Geometry check sheet. Reference: the model listing, model coordinates, mm. Give positions to 0.01 mm unless a question says otherwise; leave off trailing zeros. Answer as CSV lines item,"result".
from build123d import *

# Parameters (mm, degrees)
F0_W     = 1240
F0_H     = 655
F0_W_2   = 1200
F0_H_2   = 600
F1_DEPTH = 40
F3_DEPTH = 600
F4_R     = 7.5
F5_DEPTH = 600
F6_W     = 1240
F6_H     = 655
F6_W_2   = 1200
F6_H_2   = 600
F7_DEPTH = 40


with BuildPart() as f1:
    # F0 (on Top) → F1 (new body)
    with BuildSketch(Plane.XY):
        Rectangle(F0_W, F0_H)
        Rectangle(F0_W_2, F0_H_2, mode=Mode.SUBTRACT)
    extrude(amount=F1_DEPTH)

    # F2 (on face) → F3 (join)
    with BuildSketch(Plane.XY.offset(40)):
        Polygon((-600, 327.5), (-620, 327.5), (-620, 277.5), (-600, 277.5), (-600, 300), align=None)
        Polygon((-600, -277.5), (-620, -277.5), (-620, -327.5), (-600, -327.5), (-600, -300), align=None)
        Polygon((620, 327.5), (600, 327.5), (600, 300), (600, 277.5), (620, 277.5), align=None)
        Polygon((620, -277.5), (600, -277.5), (600, -300), (600, -327.5), (620, -327.5), align=None)
    extrude(amount=F3_DEPTH)

    # F4 (on face) → F5 (join)
    with BuildSketch(Plane.XY.offset(40)):
        with Locations((-550, -315)):
            Circle(F4_R)
        with Locations((-500, -315)):
            Circle(F4_R)
        with Locations((-450, -315)):
            Circle(F4_R)
        with Locations((-400, -315)):
            Circle(F4_R)
        with Locations((-350, -315)):
            Circle(F4_R)
        with Locations((-300, -315)):
            Circle(F4_R)
        with Locations((-250, -315)):
            Circle(F4_R)
        with Locations((-200, -315)):
            Circle(F4_R)
        with Locations((-150, -315)):
            Circle(F4_R)
        with Locations((-100, -315)):
            Circle(F4_R)
        with Locations((-50, -315)):
            Circle(F4_R)
        with Locations((0, -315)):
            Circle(F4_R)
        with Locations((50, -315)):
            Circle(F4_R)
        with Locations((100, -315)):
            Circle(F4_R)
        with Locations((150, -315)):
            Circle(F4_R)
        with Locations((200, -315)):
            Circle(F4_R)
        with Locations((250, -315)):
            Circle(F4_R)
        with Locations((300, -315)):
            Circle(F4_R)
        with Locations((350, -315)):
            Circle(F4_R)
        with Locations((400, -315)):
            Circle(F4_R)
        with Locations((450, -315)):
            Circle(F4_R)
        with Locations((500, -315)):
            Circle(F4_R)
        with Locations((550, -315)):
            Circle(F4_R)
        with Locations((-500, 315)):
            Circle(F4_R)
        with Locations((-550, 315)):
            Circle(F4_R)
        with Locations((150, 315)):
            Circle(F4_R)
        with Locations((0, 315)):
            Circle(F4_R)
        with Locations((250, 315)):
            Circle(F4_R)
        with Locations((-400, 315)):
            Circle(F4_R)
        with Locations((450, 315)):
            Circle(F4_R)
        with Locations((100, 315)):
            Circle(F4_R)
        with Locations((500, 315)):
            Circle(F4_R)
        with Locations((-100, 315)):
            Circle(F4_R)
        with Locations((-450, 315)):
            Circle(F4_R)
        with Locations((400, 315)):
            Circle(F4_R)
        with Locations((50, 315)):
            Circle(F4_R)
        with Locations((-300, 315)):
            Circle(F4_R)
        with Locations((-50, 315)):
            Circle(F4_R)
        with Locations((550, 315)):
            Circle(F4_R)
        with Locations((300, 315)):
            Circle(F4_R)
        with Locations((-200, 315)):
            Circle(F4_R)
        with Locations((200, 315)):
            Circle(F4_R)
        with Locations((350, 315)):
            Circle(F4_R)
        with Locations((-250, 315)):
            Circle(F4_R)
        with Locations((-150, 315)):
            Circle(F4_R)
        with Locations((-350, 315)):
            Circle(F4_R)
        with Locations((-610, -263.75)):
            Circle(F4_R)
        with Locations((-610, -213.75)):
            Circle(F4_R)
        with Locations((-610, -163.75)):
            Circle(F4_R)
        with Locations((-610, -113.75)):
            Circle(F4_R)
        with Locations((-610, -63.75)):
            Circle(F4_R)
        with Locations((-610, -13.75)):
            Circle(F4_R)
        with Locations((-610, 36.25)):
            Circle(F4_R)
        with Locations((-610, 86.25)):
            Circle(F4_R)
        with Locations((-610, 136.25)):
            Circle(F4_R)
        with Locations((-610, 186.25)):
            Circle(F4_R)
        with Locations((-610, 236.25)):
            Circle(F4_R)
        with Locations((610, -263.75)):
            Circle(F4_R)
        with Locations((610, -213.75)):
            Circle(F4_R)
        with Locations((610, 136.25)):
            Circle(F4_R)
        with Locations((610, 236.25)):
            Circle(F4_R)
        with Locations((610, -113.75)):
            Circle(F4_R)
        with Locations((610, 86.25)):
            Circle(F4_R)
        with Locations((610, 186.25)):
            Circle(F4_R)
        with Locations((610, 36.25)):
            Circle(F4_R)
        with Locations((610, -13.75)):
            Circle(F4_R)
        with Locations((610, -63.75)):
            Circle(F4_R)
        with Locations((610, -163.75)):
            Circle(F4_R)
    extrude(amount=F5_DEPTH)

    # F6 (on face) → F7 (join)
    with BuildSketch(Plane.XY.offset(640)):
        Rectangle(F6_W, F6_H)
        Rectangle(F6_W_2, F6_H_2, mode=Mode.SUBTRACT)
    extrude(amount=F7_DEPTH)


solid = f1.part
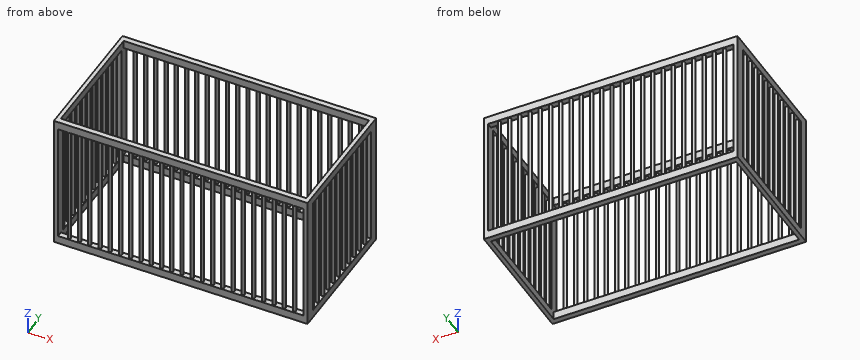
(1) Material ranges on line 1 (Y direction, x = 1.5, z = 130); line 2 (Y direction, x = 145, z = 653.5); line 3 (X direction, y = -287.5, z = 560.5), recorded low to high.
The answers:
line 1,"y = -322.35 to -307.65, 307.65 to 322.35"
line 2,"y = -327.5 to -300, 300 to 327.5"
line 3,"x = -620 to -600, 600 to 620"
(2) Section check A-A on z = 380.5. State how many separate pieces and enclosed holes the cut face has, then the cut area to 3 significant figures.
The answers:
separate pieces,"72"
enclosed holes,"0"
area,"16,000 mm2"
(3) Gauge pin test, flat ends, axial feed: P1, Ø8, axis at y = 182.5, z = 220.5, coming from the -X side; P2, Ø6, axis at x = -605.5, y = 1, coming from the -Z side. Record the tip position at first contact, or that the pin passes through.
The answers:
P1,"stops at x = -617.5"
P2,"stops at z = 0"
